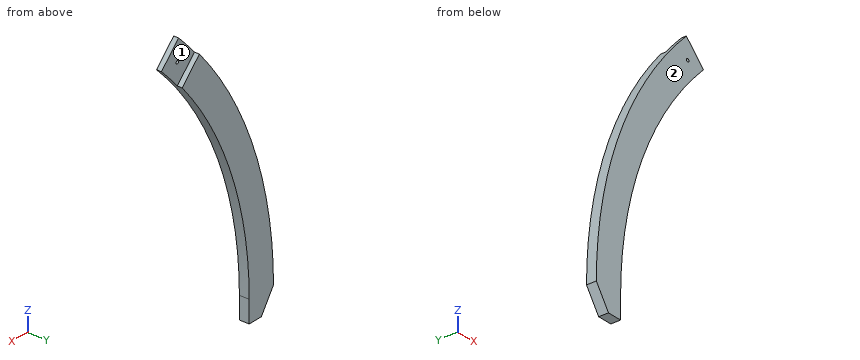
Autodesk Inventor part; units mm, degrees
ref_plane "YZ Plane" through (0, 0, 0) normal (1, 0, 0) x (0, 1, 0)
ref_plane "XZ Plane" through (0, 0, 0) normal (0, 1, 0) x (-1, 0, 0)
ref_plane "XY Plane" through (0, 0, 0) normal (0, 0, 1) x (1, 0, 0)
sketch "Sketch1" plane through (0, 0, 0) normal (0, 1, 0) x (-1, 0, 0)
  arc A0 (350, 0) -> (0, 350) centre (0, 0) ccw
  line L0 (350, 0) -> (350, -22.2048)
  line L1 (0, 350) -> (-24.6, 350)
  line L2 (-24.6, 380) -> (0, 380)
  arc A1 (380, 0) -> (0, 380) centre (0, 0) ccw
  line L3 (380, 0) -> (380, -22.2048)
  line L4 (380, -22.2048) -> (350, -22.2048)
  line L5 (-24.6, 380) -> (-24.6, 350)
  line L6 (380, 0) -> (365, -22.2048)
  line L7 (0, 0) -> (268.7006, 268.7006)
  line L8 (0, 0) -> (0, 91.6225)
  point P0 (247.4874, 247.4874)
  dimension "d0" = 350
  dimension "d1" = 374.6
  dimension "d2" = 30
extrude "Extrusion1" add sketch "Sketch1" along normal blind 10 contours A0 L7 A1 L6 L4 L0
sketch "Sketch2" plane through (0, 10, 0) normal (0, 1, 0) x (1, 0, 0)
  line L0 (-350, 22.2048) -> (-365, 22.2048)
  line L1 (-365, 22.2048) -> (-380, 0)
  arc A0 (-380, 0) -> (-268.7006, -268.7006) centre (0, 0) ccw
  line L2 (-268.7006, -268.7006) -> (-247.4874, -247.4874)
  arc A1 (-350, 0) -> (-247.4874, -247.4874) centre (0, 0) ccw
  line L3 (-350, 0) -> (-350, 22.2048)
  line L4 (-288.3574, -247.4874) -> (-267.0773, -226.2072)
extrude "Extrusion2" cut sketch "Sketch2" against normal blind 5 contours A1 L2 A0 L4
sketch "Sketch3" plane through (0, 10, 0) normal (0, 1, 0) x (1, 0, 0)
  arc A0 (-267.0773, -226.2072) -> (-247.4874, -247.4874) centre (0, 0) ccw
  line L0 (-288.3574, -247.4874) -> (-267.0773, -226.2072)
  arc A1 (-288.3574, -247.4874) -> (-268.7006, -268.7006) centre (0, 0) ccw
  line L1 (-247.4874, -247.4874) -> (-268.7006, -268.7006)
  circle A2 centre (-267.0773, -247.4874) radius 1.55
  dimension "d7" = 3.1
extrude "Extrusion3" cut sketch "Sketch3" against normal through all contours A2
properties part number "MOLDE_CURVA_1" material "Steel, Mild, Welded"
CAD build for the part. Positions are in the model's coordinates, mm. Face numbers are marked on the shaded views. A direction names the side the tool comes from. Round coordinates to 2 decimals unless told otherwise and drop trailing zeros. Order: outer loops, then holes, each group sorted by start corner. A loop starts at its lowest first (then second) coordinate and runs counter-clockwise, first axis right, second up.
Item 1: Tool access for the marked faces 1 and 2: list every direction of +Z, -Z, +X, -X, +Y, -Y with a clear straight run to the whole face (end or side of a thin tool).
Item 2: Saw through at A-A on y = 1.75. Write the cut outline in (x, z), then the cut area to 3 significant figures.
Item 3: Saw through at B-B on x = -331. Write the cut outline in (y, z).
Item 4: Saw through at C-C on z = 117. Write the cut outline in (x, y).
Item 5: Probe line 1 along X through (y, z) = (1.25, 4); line 2 along X through (y, z) = (7, 204); line 3 along Z through (x, y) = (-322, 3). List the from-to ranges inside material, lowest first.
Item 6: Pin check, flat tip, straight feed: pin 1 (3 mm diameter, centred on y = 8, z = 28, fed in from +X). Stop position of the tip, or through.
Item 7: Saw through at D-D on z = 237. Write the cut outline in (x, y), then the cut area to 3 significant figures.
Reported:
1. face 1: +Z, +X, +Y
1. face 2: +Z, -Z, +X, -X, -Y
2. outline: (-380, 0) - (-365, -22.2) - (-350, -22.2) - (-350, 0) arc R350 cw to (-247.49, 247.49) - (-268.7, 268.7) arc R380 ccw to start; hole circle Ø3.1 at (-267.08, 247.49)
2. area: 9,090 mm2
3. outline: (0, 113.75) - (10, 113.75) - (10, 186.65) - (0, 186.65) - close
4. outline: (-361.54, 0) - (-329.87, 0) - (-329.87, 10) - (-361.54, 10) - close
5. line 1: x = -379.98 to -349.98
5. line 2: x = -320.6 to -284.4
5. line 3: z = 137.17 to 201.78
6. pin 1: stops at x = -348.75
7. outline: (-297.04, 0) - (-257.55, 0) - (-257.55, 5) - (-277.87, 5) - (-277.87, 10) - (-297.04, 10) - close
7. area: 293 mm2
